Read the model definition and answer for the solid it produces. Units are mm, in the model's axes. A direction names the side the tool comes from. Coordinates: 2 decimals unless noted, no trailing zeros. Write each loop counter-clockwise with the first axis right and the second up, starting at its lowest first coordinate (ties: lowest second). Pieces come first, ordered by that corner, then holes. Notation, with made-up numbers: (66, 9) -> (76, 9) arc R24 ccw to (76, 25) -> close; hole circle Ø6 at (33.5, 33). An arc over 180 degrees is marked (long way). Use CSV: the item, a comma, the result in double quotes. Start each with the question number.
from build123d import *

# Parameters (mm, degrees)
F1_DEPTH       = 16
F2_W           = 20
F2_H           = 76
F2_W_2         = 16
F2_H_2         = 20
F3_DEPTH       = 16
F4_R           = 10
F6_D           = 3.3
F6_CSINK_D     = 6.72
F6_CSINK_ANGLE = 90
F8_D           = 6.6
F8_DEPTH       = 30
F8_TIP         = 1.9828400428
F10_D          = 4.4
F12_D          = 3.3


with BuildPart() as f1:
    # F0 (on Top) → F1 (new body)
    with BuildSketch(Plane.XY):
        Polygon((195, -220), (195, 220), (-195, 220), (-195, -220), (-135, -220), (-135, 160), (135, 160), (135, -220), align=None)
    extrude(amount=F1_DEPTH)

    # F2 (on face) → F3 (cut, through all)
    with BuildSketch(Plane.XY.offset(16)):
        with Locations((-145, -182)):
            Rectangle(F2_W, F2_H)
        with Locations((-165, 166)):
            Rectangle(F2_W_2, F2_H_2)
        with Locations((-165, -114)):
            Rectangle(F2_W_2, F2_H_2)
        with Locations((-165, 26)):
            Rectangle(F2_W_2, F2_H_2)
        with Locations((145, -182)):
            Rectangle(F2_W, F2_H)
        with Locations((165, 26)):
            Rectangle(F2_W_2, F2_H_2)
        with Locations((165, 166)):
            Rectangle(F2_W_2, F2_H_2)
        with Locations((165, -114)):
            Rectangle(F2_W_2, F2_H_2)
    extrude(amount=-F3_DEPTH, mode=Mode.SUBTRACT)

    # F4
    f4_edges = [f1.edges().sort_by_distance(p)[0] for p in [
        (-135, 160, 8),
        (135, 160, 8),
        (-195, 220, 8),
        (195, 220, 8),
        (195, -220, 8),
        (155, -220, 8),
        (-155, -220, 8),
        (-195, -220, 8),
    ]]
    fillet(f4_edges, radius=F4_R)

    # F6 (through all)
    with Locations(Plane.XY.offset(16)):
        with Locations((-165, 96), (-165, -44), (165, 96), (165, -44)):
            CounterSinkHole(F6_D / 2, F6_CSINK_D / 2, counter_sink_angle=F6_CSINK_ANGLE)

    # F8
    with Locations(Plane.XZ.offset(220)):
        with Locations((-175, 8), (175, 8)):
            Hole(F8_D / 2, depth=F8_DEPTH)
            with Locations((0, 0, -(F8_DEPTH + F8_TIP / 2))):  # 118° drill point
                Cone(0, F8_D / 2, F8_TIP, mode=Mode.SUBTRACT)

    # F10 (through all)
    with Locations(Plane.XY.offset(16)):
        with Locations((-187, 201), (-153, 201), (187, 201), (153, 201)):
            Hole(F10_D / 2)

    # F12 (through all)
    with Locations(Plane.XY.offset(16)):
        with Locations((-186.5, -168.75), (-186.5, -211.25), (186.5, -211.25), (186.5, -168.75)):
            Hole(F12_D / 2)


solid = f1.part
1) Find the intervals of material crossed by line 1 along X through (y, z) = (171.5, 9); line 2 along X through (y, z) = (-44, 8.5); line 3 along X through (y, z) = (-168.75, 8), in increasing order.
2) Section A-A, the plane y = -131.5 is taken. Give the vertices of the cut face in (x, z), plus the area to 3 significant figures.
3) Which of the six approach directions +Z, -Z, +X, -X, +Y, -Y give full straight-line access (tool end or side, diameter ignored) to faces 5 (the face through (-175, -220, 4)), 6 (the face through (-145, -144, 8)), 7 (the face through (165, 16, 8))?
4) Section B-B, the plane x = -53 is taken. Give the vertices of the cut face in (y, z), plus the area to 3 significant figures.
5) The mould has two halves that part along X. Classify faces 1 (the face through (-195, 3, 8)), 2 (the face through (145, -144, 8)), 3 (the face through (3, 220, 8)), 4 (the face through (-165, 36, 8)): pulls with the +X half, pulls with the -X half, needs draft (parallel to the pull), parting line crosses it, or undercut.
6) Each of these flat-tipped pins is pushed along its axis until it touches: pin 1 (4 mm diameter, centred on x = 186.5, y = -168.75, fed in from -Z); pin 2 (5 mm diameter, centred on x = -96, z = 3, fed in from -Y). Where does it stop, or does it pass through?
The answers:
1,line 1,"x = -195 to -173, -157 to 157, 173 to 195"
1,line 2,"x = -195 to -166.65, -163.35 to -135, 135 to 163.35, 166.65 to 195"
1,line 3,"x = -195 to -188.15, -184.85 to -155, 155 to 184.85, 188.15 to 195"
2,outline,"(-195, 0) -> (-135, 0) -> (-135, 16) -> (-195, 16) -> close; (135, 0) -> (195, 0) -> (195, 16) -> (135, 16) -> close"
2,area,"1,920 mm^2"
3,face 5,"+Z, -Z, +X, -X, -Y"
3,face 6,"+Z, -Z, -Y"
3,face 7,"+Z, -Z"
4,outline,"(160, 0) -> (220, 0) -> (220, 16) -> (160, 16) -> close"
4,area,"960 mm^2"
5,face 1,"pulls with the -X half"
5,face 2,"undercut"
5,face 3,"needs draft"
5,face 4,"undercut"
6,pin 1,"stops at z = 0"
6,pin 2,"stops at y = 160"
